Read the model definition and answer for the solid it produces. Units are mm, in the model's axes. Face numbers are marked on the shaded views. Coordinates: 2 decimals unless noted, no trailing zeros. Write each loop counter-clockwise with the first axis right and the second up, starting at its lowest first coordinate (ties: lowest second). Pieces come first, ordered by that corner, then holes. Notation, with made-up numbers: (88, 35.25) -> (131, 35.25) arc R27 ccw to (131, 71.25) -> close; hole circle Ø2 at (10, 59.5). An arc over 180 degrees is marked (long way). Use CSV: the item, a comma, the result in double quotes.
from build123d import *

# Parameters (mm, degrees)
SKETCH1_R                = 59
EXTRUDE1_DEPTH           = 3
EXTRUDE2_DEPTH           = 3
CIRPATTERN1_COUNT        = 6
F_2_0_2_DIAMETER_HOLE1_D = 2
F_2_0_2_DIAMETER_HOLE3_D = 2
F_2_0_2_DIAMETER_HOLE4_D = 2
CIRPATTERN2_COUNT        = 6
CIRPATTERN3_COUNT        = 6


with BuildPart() as part:
    # Sketch1 → Extrude1 (new, symmetric)
    with BuildSketch(Plane(origin=(0, 0, 0), x_dir=(0, 0, -1), z_dir=(1, 0, 0))):
        Circle(SKETCH1_R)
        Polygon((28.815179183, 2.521001516), (12.224338236, 26.215177945), (-16.590840947, 23.694176429), (-28.815179183, -2.521001516), (-12.224338236, -26.215177945), (16.590840947, -23.694176429), align=None, mode=Mode.SUBTRACT)
    extrude(amount=EXTRUDE1_DEPTH, both=True)

    # Sketch2 → Extrude2 (add, symmetric)
    with BuildSketch(Plane(origin=(0, 0, 0), x_dir=(0, 0, -1), z_dir=(1, 0, 0))):
        with BuildLine():
            Line((-2, 67.961805723), (-0.262709442, 61.478149092))
            ThreePointArc((-0.262709442, 61.478149092), (-0.58620663, 59.77173183), (-2.122608272, 58.961805723))
            ThreePointArc((-2.122608272, 58.961805723), (28.679663449, 51.560419941), (51.21368579, 29.294340542))
            ThreePointArc((51.21368579, 29.294340542), (36.791707484, 48.186627241), (17.927108603, 62.644803614))
            ThreePointArc((17.927108603, 62.644803614), (8.312130826, 66.609702921), (-2, 67.961805723))
        make_face()
    extrude2 = extrude(amount=EXTRUDE2_DEPTH, both=True)

    # CirPattern1: Extrude2 ×6 about axis
    cirpattern1_axis = Axis((0, 0, 0), (1, 0, 0))
    for i in range(1, CIRPATTERN1_COUNT):
        add(extrude2.rotate(cirpattern1_axis, i * 360 / CIRPATTERN1_COUNT))

    # Ø2.0 (2) Diameter Hole1 (through all)
    with Locations(Plane(origin=(3, 0, 0), x_dir=(0, 0, -1), z_dir=(1, 0, 0))):
        with Locations((12.224338236, 26.215177945), (28.815179183, 2.521001516), (16.590840947, -23.694176429), (-12.224338236, -26.215177945), (-28.815179183, -2.521001516), (-16.590840947, 23.694176429)):
            Hole(F_2_0_2_DIAMETER_HOLE1_D / 2)

    # Ø2.0 (2) Diameter Hole3 (through all)
    with Locations(Plane(origin=(3, 0, 0), x_dir=(0, 0, -1), z_dir=(1, 0, 0))):
        with Locations((17.945810697, 18.044068454)):
            f_2_0_2_diameter_hole3 = Hole(F_2_0_2_DIAMETER_HOLE3_D / 2)

    # Ø2.0 (2) Diameter Hole4 (through all)
    with Locations(Plane(origin=(3, 0, 0), x_dir=(0, 0, -1), z_dir=(1, 0, 0))):
        with Locations((23.38049494, 10.282534985)):
            f_2_0_2_diameter_hole4 = Hole(F_2_0_2_DIAMETER_HOLE4_D / 2)

    # CirPattern2: Ø2.0 (2) Diameter Hole3 ×6 about axis
    cirpattern2_axis = Axis((0, 0, 0), (1, 0, 0))
    for i in range(1, CIRPATTERN2_COUNT):
        add(f_2_0_2_diameter_hole3.rotate(cirpattern2_axis, i * 360 / CIRPATTERN2_COUNT), mode=Mode.SUBTRACT)

    # CirPattern3: Ø2.0 (2) Diameter Hole4 ×6 about axis
    cirpattern3_axis = Axis((0, 0, 0), (1, 0, 0))
    for i in range(1, CIRPATTERN3_COUNT):
        add(f_2_0_2_diameter_hole4.rotate(cirpattern3_axis, i * 360 / CIRPATTERN3_COUNT), mode=Mode.SUBTRACT)


solid = part.part
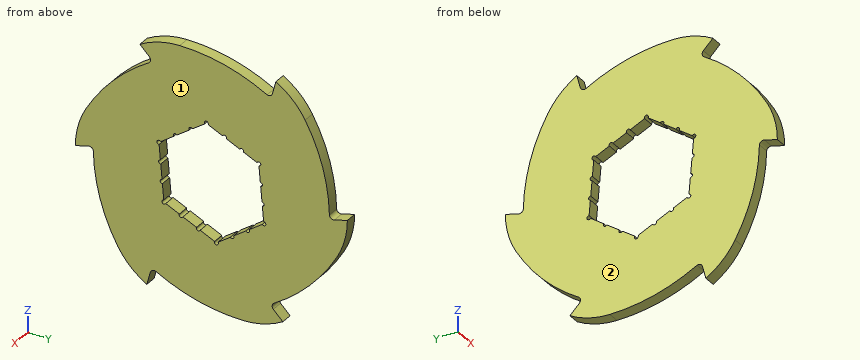
1. Each of these flat-tipped pins is pushed along its axis until it touches: pin 1 Ø3 at (x, y) = (0.5, 33.5) entering from -Z; pin 2 Ø3 at (x, z) = (1, 13) entering from +Y; pin 3 Ø1.6 at (y, z) = (-23.69, -16.59) entering from -X. Where does it stop, or does it pass through?
Solutions:
pin 1,"stops at z = -59.75"
pin 2,"stops at y = 58.28"
pin 3,"passes through"
2. A cutting plane is placed at C-C (z = 38). Give the vertices of the cut face in (x, y), and give its area (3 significant figures).
Solutions:
outline,"(-3, -46.95) -> (3, -46.95) -> (3, 50.64) -> (-3, 50.64) -> close"
area,"586 mm^2"
3. For a pull along X with two mould halves and no side action, classify the marked faces 1 and 2 as pulls with the +X half, pulls with the -X half, needs draft (parallel to the pull), parting line crosses it, or undercut.
Solutions:
face 1,"pulls with the +X half"
face 2,"pulls with the -X half"
4. Find the intervals of material crossed by line 1 along Z through (x, y) = (2, 35.5); line 2 along Y through (x, z) = (0.85, 4); line 3 along Z through (x, y) = (-1, 12.5), in increasing order.
Solutions:
line 1,"z = -57.98 to -57.64, -47.32 to 57.76"
line 2,"y = -67.51 to -25.5, 24.8 to 58.92"
line 3,"z = -63.16 to -21.83, 21.81 to 58.71"
5. A cutting plane is placed at A-A (z = -55). Give the vertices of the cut face in (x, y), and give its area (3 significant figures).
Solutions:
outline,"(-3, -38.95) -> (3, -38.95) -> (3, -30.95) -> (-3, -30.95) -> close; (-3, -21.96) -> (3, -21.96) -> (3, 32.86) -> (-3, 32.86) -> close"
area,"377 mm^2"
6. A cutting plane is placed at B-B (y = -51). Give the vertices of the cut face in (x, z), and give its area (3 significant figures).
Solutions:
outline,"(-3, -37.22) -> (3, -37.22) -> (3, 33.85) -> (-3, 33.85) -> close"
area,"426 mm^2"
